The listing builds one solid part. Answer for the finished solid, in the listing's coordinates (mm). Give positions to 0.01 mm unless a question says otherwise; leave off trailing zeros. Loops run counter-clockwise (first coordinate to the right, second up) from the corner with the lowest first, then second, coordinate; pieces in that order, holes last. Notation, with made-up numbers: (22.5, 51) - (62.5, 51) arc R18 ccw to (62.5, 61) - close; hole circle Ø3 at (-13.75, 83.5). An arc over 180 degrees is marked (long way). Answer as CSV lines item,"result". Start each with the question number.
1) A cutting plane is placed at C-C (z = -1). Determine the outline of the cut face in (x, y), and give its area (3 significant figures).
2) Find the intervals of material crossed by line 1 along Y through (x, z) = (0, -2.5); line 2 along Y through (x, z) = (-14, -1.5); line 3 along X through (y, z) = (-3, -1.5), in increasing order.
3) A flat-ended cylindrical pin translates along its axis: pin 1 (3 mm diameter, centred on x = 46, y = -3.5, fed in from +Z). Find the tip coordinate at first contact, or state that the pin passes through.
4) For a pull along X with two mould halves and no side action, classify faces 1 (the face through (-30.235, -23.183, -3.131)), 2 (the face through (63.5, -1, -3)), 3 (the face through (-63.5, 1, -3)), 4 (the face through (-6, 38, 0)) as pulls with the +X half, pulls with the -X half, needs draft (parallel to the pull), parting line crosses it, or undercut.
5) A cutting plane is placed at A-A (y = 0). Determine the outline of the cut face in (x, z).
Autodesk Inventor part; units mm, degrees
ref_plane "YZ Plane" through (0, 0, 0) normal (1, 0, 0) x (0, 1, 0)
ref_plane "XZ Plane" through (0, 0, 0) normal (0, 1, 0) x (-1, 0, 0)
ref_plane "XY Plane" through (0, 0, 0) normal (0, 0, 1) x (1, 0, 0)
sketch "Sketch1" plane through (0, 0, 0) normal (0, 0, 1) x (1, 0, 0)
  circle A0 centre (0, 0) radius 48.5902 construction
  circle A1 centre (0, 0) radius 42.1132 construction
  circle A2 centre (0, 0) radius 54.61 construction
  circle A3 centre (0, 0) radius 51.7652 construction
  line L0 (0, 0) -> (0, 45.3517) construction
  circle A4 centre (0, 0) radius 38.1
  line L1 (-63.5, -63.5) -> (63.5, -63.5)
  line L2 (63.5, -63.5) -> (63.5, 63.5)
  line L3 (63.5, 63.5) -> (-63.5, 63.5)
  line L4 (-63.5, 63.5) -> (-63.5, -63.5)
  line L5 (-63.5, -63.5) -> (63.5, 63.5) construction
  line L6 (63.5, -63.5) -> (-63.5, 63.5) construction
  dimension "d0" = 97.1804
  dimension "d1" = 84.2264
  dimension "d2" = 109.22
  dimension "d3" = 103.5304
  dimension "d15" = 45.3517
  dimension "d27" = 76.2
  dimension "d28" = 127
  dimension "d29" = 127
sketch "Sketch2" plane through (0, 0, 0) normal (1, 0, 0) x (0, 1, 0)
  line L0 (0, 0) -> (45.3517, 0) construction
  line L1 (45.3517, 0) -> (45.3517, 0.7937) construction
  circle A0 centre (45.3517, 0.7937) radius 3.2385
  line L2 (0, 0) -> (0, 25.4) construction
  dimension "d16" = 6.477
  dimension "d17" = 0.7937
  dimension "d18" = 25.4
extrude "Extrusion2" add sketch "Sketch1" against normal blind 6.35
revolve "Revolution2" cut sketch "Sketch2" angle 360 about axis through (0, 0, 0) along (0, 0, 1)
equation "\"d15\" = 0.25 * d1 + 0.25 * d0"
properties part number "Upper Plate" material "Aluminum 6061"
Ans:
1,outline,"(-63.5, -63.5) - (63.5, -63.5) - (63.5, 63.5) - (-63.5, 63.5) - close; circle Ø85.31 at (0, 0); hole circle Ø96.1 at (0, 0); hole circle Ø76.2 at (0, 0)"
1,area,"10,000 mm2"
2,line 1,"-63.5 to -38.1, 38.1 to 63.5"
2,line 2,"-63.5 to -45.53, -40.73 to -35.43, 35.43 to 40.73, 45.53 to 63.5"
2,line 3,"-63.5 to -47.54, -42.96 to -37.98, 37.98 to 42.96, 47.54 to 63.5"
3,pin 1,"z = -1.5"
4,face 1,"undercut"
4,face 2,"pulls with the +X half"
4,face 3,"pulls with the -X half"
4,face 4,"needs draft"
5,outline,"(-63.5, -6.35) - (-38.1, -6.35) - (-38.1, 0) - (-42.21, 0) arc R3.24 cw to (-48.49, 0) - (-63.5, 0) - close; (38.1, -6.35) - (63.5, -6.35) - (63.5, 0) - (48.49, 0) arc R3.24 cw to (42.21, 0) - (38.1, 0) - close"
